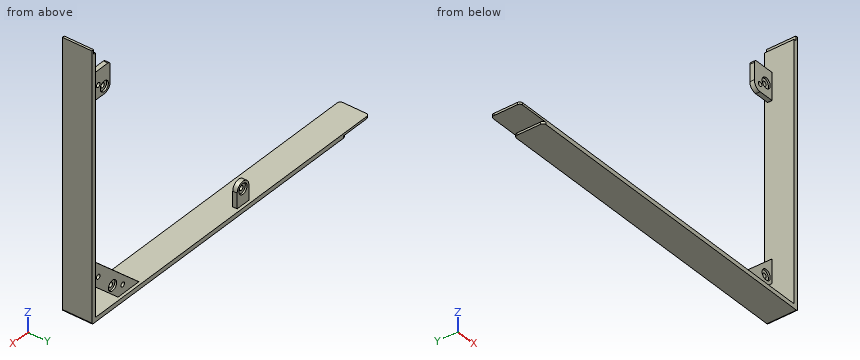
from build123d import *

# Parameters (mm, degrees)
EXTRUDE_1_DEPTH     = 20
EXTRUDE_START       = 1
SKETCH_2_R          = 1.525
EXTRUDE_2_DEPTH     = 3
CUT_EXTRUDE_1_REACH = 358.708
SKETCH_3_W          = 31
SKETCH_3_H          = 9.5
SKETCH_4_R          = 3.5
CUT_EXTRUDE_2_DEPTH = 1.2
CUT_EXTRUDE_3_REACH = 356.959
SKETCH_5_R          = 1.525
FILLET_1_R          = 1
FILLET_3_R          = 1
SKETCH_6_R          = 3.5
CUT_EXTRUDE_4_DEPTH = 1.2
SKETCH_7_W          = 69.4
SKETCH_7_H          = 20
CUT_EXTRUDE_5_DEPTH = 3
SKETCH_8_W          = 20
SKETCH_8_H          = 20
CUT_EXTRUDE_6_DEPTH = 1.5
FILLET_4_R          = 2
FILLET_5_R          = 2
FILLET_6_R          = 2


with BuildPart() as part:
    # 草图1 → 凸台-拉伸1 (new body)
    with BuildSketch(Plane(origin=(0, 0, 0), x_dir=(1, 0, 0), z_dir=(0, 1, 0))):
        Polygon((1.5, 0), (3, 0), (3, 173.85), (307.4, 173.85), (307.4, 176.85), (0, 176.85), (0, 0), (0, -3), (1.5, -3), align=None)
    extrude(amount=EXTRUDE_1_DEPTH)

    # 草图2 → 凸台-拉伸2 (add)
    # profile 1 of 3: a face of its own
    with BuildSketch(Plane(origin=(0, 14, 0), x_dir=(1, 0, 0), z_dir=(0, 1, 0)).offset(EXTRUDE_START)):
        Polygon((3, 153.85), (25, 173.85), (42.839282497, 173.85), (3, 137.632470457), align=None)
        with Locations(Location((20.25, 163.5, 0), (0, 0, 270))):
            Circle(SKETCH_2_R, mode=Mode.SUBTRACT)
    # profile 2 of 3: a face of its own
    with BuildSketch(Plane(origin=(0, 14, 0), x_dir=(1, 0, 0), z_dir=(0, 1, 0)).offset(EXTRUDE_START)):
        with BuildLine():
            Line((137.25, 163.5), (137.25, 173.85))
            Line((137.25, 173.85), (127.25, 173.85))
            Line((127.25, 173.85), (127.25, 163.5))
            ThreePointArc((127.25, 163.5), (132.25, 158.5), (137.25, 163.5))
        make_face()
        with Locations(Location((132.25, 163.5, 0), (0, 0, 270))):
            Circle(SKETCH_2_R, mode=Mode.SUBTRACT)
    # profile 3 of 3: a face of its own
    with BuildSketch(Plane(origin=(0, 14, 0), x_dir=(1, 0, 0), z_dir=(0, 1, 0)).offset(EXTRUDE_START)):
        with BuildLine():
            Line((3, 23.870342351), (3, 33.5))
            Line((3, 33.5), (13.2, 33.5))
            ThreePointArc((13.2, 33.5), (16.735533906, 32.035533906), (18.2, 28.5))
            Line((18.2, 28.5), (18.2, 15.043961292))
            Line((18.2, 15.043961292), (3, 15.043961292))
            Line((3, 15.043961292), (3, 23.870342351))
        make_face()
        with Locations(Location((13.2, 28.5, 0), (0, 0, 270))):
            Circle(SKETCH_2_R, mode=Mode.SUBTRACT)
    extrude(amount=EXTRUDE_2_DEPTH)

    # 草图3 → 切除-拉伸1 (cut, up to next)
    with BuildSketch(Plane(origin=(0, 0, -176.85), x_dir=(-1, 0, 0), z_dir=(0, 0, -1)), mode=Mode.PRIVATE) as cut_extrude_1_sk1:
        with Locations((-291.9, 15.25)):
            Rectangle(SKETCH_3_W, SKETCH_3_H)
    cut_extrude_1_tool1 = extrude(cut_extrude_1_sk1.sketch, amount=-CUT_EXTRUDE_1_REACH, mode=Mode.PRIVATE) & part.part
    add(cut_extrude_1_tool1.solids().sort_by_distance((291.9, 15.25, -176.85))[0], mode=Mode.SUBTRACT)

    # 草图4 → 切除-拉伸2 (cut)
    with BuildSketch(Plane(origin=(0, 18, 0), x_dir=(1, 0, 0), z_dir=(0, 1, 0))):
        with Locations(Location((13.2, 28.5, 0), (0, 0, 270))):
            Circle(SKETCH_4_R)
        with Locations(Location((20.25, 163.5, 0), (0, 0, 270))):
            Circle(SKETCH_4_R)
        with Locations(Location((132.25, 163.5, 0), (0, 0, 270))):
            Circle(SKETCH_4_R)
    extrude(amount=-CUT_EXTRUDE_2_DEPTH, mode=Mode.SUBTRACT)

    # 草图5 → 切除-拉伸3 (cut, up to next)
    with BuildSketch(Plane.XZ.offset(-15), mode=Mode.PRIVATE) as cut_extrude_3_sk1:
        with Locations(Location((29, -167.85, 0), (0, 0, 270))):
            Circle(SKETCH_5_R)
    cut_extrude_3_tool1 = extrude(cut_extrude_3_sk1.sketch, amount=-CUT_EXTRUDE_3_REACH, mode=Mode.PRIVATE) & part.part
    # 草图5 → 切除-拉伸3 (cut, up to next)
    with BuildSketch(Plane.XZ.offset(-15), mode=Mode.PRIVATE) as cut_extrude_3_sk2:
        with Locations(Location((8, -150.85, 0), (0, 0, 270))):
            Circle(SKETCH_5_R)
    cut_extrude_3_tool2 = extrude(cut_extrude_3_sk2.sketch, amount=-CUT_EXTRUDE_3_REACH, mode=Mode.PRIVATE) & part.part
    # 草图5 → 切除-拉伸3 (cut, up to next)
    with BuildSketch(Plane.XZ.offset(-15), mode=Mode.PRIVATE) as cut_extrude_3_sk3:
        with Locations(Location((8, -24.8, 0), (0, 0, 270))):
            Circle(SKETCH_5_R)
    cut_extrude_3_tool3 = extrude(cut_extrude_3_sk3.sketch, amount=-CUT_EXTRUDE_3_REACH, mode=Mode.PRIVATE) & part.part
    add(cut_extrude_3_tool1.solids().sort_by_distance((29, 15, -167.85))[0], mode=Mode.SUBTRACT)
    add(cut_extrude_3_tool2.solids().sort_by_distance((8, 15, -150.85))[0], mode=Mode.SUBTRACT)
    add(cut_extrude_3_tool3.solids().sort_by_distance((8, 15, -24.8))[0], mode=Mode.SUBTRACT)

    # 圆角1
    fillet_1_edges = [part.edges().sort_by_distance(p)[0] for p in [
        (0, 10, -176.85),
    ]]
    fillet(fillet_1_edges, radius=FILLET_1_R)

    # 圆角3
    fillet_3_edges = [part.edges().sort_by_distance(p)[0] for p in [
        (276.4, 10.5, -175.35),
    ]]
    fillet(fillet_3_edges, radius=FILLET_3_R)

    # 草图6 → 切除-拉伸4 (cut)
    with BuildSketch(Plane.XZ.offset(-15)):
        with Locations(Location((8, -24.8, 0), (0, 0, 270))):
            Circle(SKETCH_6_R)
        with Locations(Location((8, -150.85, 0), (0, 0, 270))):
            Circle(SKETCH_6_R)
        with Locations(Location((29, -167.85, 0), (0, 0, 270))):
            Circle(SKETCH_6_R)
    extrude(amount=-CUT_EXTRUDE_4_DEPTH, mode=Mode.SUBTRACT)

    # 草图7 → 切除-拉伸5 (cut)
    with BuildSketch(Plane(origin=(0, 0, -176.85), x_dir=(-1, 0, 0), z_dir=(0, 0, -1))):
        with Locations((-272.7, 10)):
            Rectangle(SKETCH_7_W, SKETCH_7_H)
    extrude(amount=-CUT_EXTRUDE_5_DEPTH, mode=Mode.SUBTRACT)


with BuildPart() as body_2:
    # 镜向3: mirrored copy
    add(part.part.mirror(Plane(origin=(317.4, 0, 0), x_dir=(0, 0, 1), z_dir=(1, 0, 0))))

    # 草图8 → 切除-拉伸6 (cut)
    with BuildSketch(Plane(origin=(0, 0, -176.85), x_dir=(-1, 0, 0), z_dir=(0, 0, -1))):
        with Locations((-406.8, 10)):
            Rectangle(SKETCH_8_W, SKETCH_8_H)
    extrude(amount=-CUT_EXTRUDE_6_DEPTH, mode=Mode.SUBTRACT)

    # 圆角4
    fillet_4_edges = [body_2.edges().sort_by_distance(p)[0] for p in [
        (416.8, 0, -176.1),
        (416.8, 20, -176.1),
    ]]
    fillet(fillet_4_edges, radius=FILLET_4_R)

    # 圆角5
    fillet_5_edges = [body_2.edges().sort_by_distance(p)[0] for p in [
        (396.8, 20, -174.6),
        (396.8, 0, -174.6),
    ]]
    fillet(fillet_5_edges, radius=FILLET_5_R)

    # 圆角6
    fillet_6_edges = [body_2.edges().sort_by_distance(p)[0] for p in [
        (616.6, 16.5, -15.043961292),
    ]]
    fillet(fillet_6_edges, radius=FILLET_6_R)


solid = body_2.part
Source: CAD feature listing. Evaluate the final solid. Frame: model axes, mm. Give positions to 0.01 mm unless a question says otherwise; leave off trailing zeros. Order: outer loops, then holes, each group sorted by start corner. A loop starts at its lowest first (then second) coordinate and runs counter-clockwise, first axis right, second up. Notation, with made-up numbers: (70.5, -27.5) -> (89.5, -27.5) arc R16 ccw to (89.5, -5.5) -> close; hole circle Ø9 at (61.25, 45.5). An arc over 180 degrees is marked (long way). Use a Markdown table: item, result.
1) Contact query for flat-ended pins moving along their axis: P1, Ø8, axis at x = 502.55, z = -163.5, coming from the -Y side; P2, Ø1.8, axis at x = 626.8, z = -24.8, coming from the -Y side; P3, Ø1, axis at y = 3, z = -95, coming from the -X side; P4, Ø12, axis at x = 623, z = -25, coming from the +Y side. Output: stop coordinate, or through.
Answer list:
| item | result |
|---|---|
| P1 | y = 15 |
| P2 | through |
| P3 | x = 631.8 |
| P4 | y = 18 |
2) Section query B-B, the plane z = -61. Return the cut outline in (x, y).
Answer list:
| item | result |
|---|---|
| outline | (631.8, 0) -> (634.8, 0) -> (634.8, 20) -> (631.8, 20) -> close |
3) Section query A-A, the plane y = 12.5. Return the cut outline in (x, z), then the cut area to 3 significant figures.
Answer list:
| item | result |
|---|---|
| outline | (396.8, -175.35) -> (416.8, -175.35) -> (416.8, -176.85) -> (633.8, -176.85) arc R1 ccw to (634.8, -175.85) -> (634.8, 3) -> (633.3, 3) -> (633.3, 0) -> (631.8, 0) -> (631.8, -173.85) -> (396.8, -173.85) -> close |
| area | 1,210 mm² |
4) Section query C-C, the plane x = 451.5. Return the cut outline in (y, z).
Answer list:
| item | result |
|---|---|
| outline | (0, -176.85) -> (20, -176.85) -> (20, -173.85) -> (0, -173.85) -> close |
5) Ray query, line 1 along Z through (x, y) = (626.8, 17.2) (3 decimals); line 2 along X through (y, z) = (16.15, -163.5) (3 decimals); line 3 along X through (y, z) = (15.8, -28.5) (3 decimals). Return the intervals inside material, ascending. Write a range as [from, to].
Answer list:
| item | result |
|---|---|
| line 1 | [-176.85, -173.85], [-158.395, -152.375], [-149.325, -142.178], [-33.5, -26.325], [-23.275, -15.044] |
| line 2 | [497.55, 501.025], [504.075, 507.55], [603.346, 613.025], [616.075, 621.185], [631.8, 634.8] |
| line 3 | [616.6, 620.075], [623.125, 634.8] |
